```python
from build123d import *

# Parameters (mm, degrees)
IZIM1_W                     = 110
IZIM1_H                     = 70
Y_KSEKLIK_EKSTR_ZYON1_DEPTH = 2
IZIM2_W                     = 110
IZIM2_H                     = 70
Y_KSEKLIK_EKSTR_ZYON2_DEPTH = 50
IZIM3_R                     = 5.5
KES_EKSTR_ZYON1_DEPTH       = 13
IZIM4_R                     = 2.5
IZIM4_W                     = 15
IZIM4_H                     = 9
KES_EKSTR_ZYON2_DEPTH       = 13
IZIM5_R                     = 1.85
KES_EKSTR_ZYON3_DEPTH       = 67


with BuildPart() as part:
    # Çizim1 → Yükseklik-Ekstrüzyon1 (new body)
    with BuildSketch(Plane(origin=(0, 0, 0), x_dir=(1, 0, 0), z_dir=(0, 1, 0))):
        Rectangle(IZIM1_W, IZIM1_H)
    extrude(amount=Y_KSEKLIK_EKSTR_ZYON1_DEPTH)

    # Çizim2 → Yükseklik-Ekstrüzyon2 (add)
    with BuildSketch(Plane(origin=(0, 2, 0), x_dir=(1, 0, 0), z_dir=(0, 1, 0))):
        Rectangle(IZIM2_W, IZIM2_H)
        with BuildLine():
            Line((-48, -33.727272727), (48, -33.727272727))
            ThreePointArc((48, -33.727272727), (49.464466094, -30.191738821), (53, -28.727272727))
            Line((53, -28.727272727), (53, 28.727272727))
            ThreePointArc((53, 28.727272727), (49.464466094, 30.191738821), (48, 33.727272727))
            Line((48, 33.727272727), (-48, 33.727272727))
            ThreePointArc((-48, 33.727272727), (-49.464466094, 30.191738821), (-53, 28.727272727))
            Line((-53, 28.727272727), (-53, -28.727272727))
            ThreePointArc((-53, -28.727272727), (-49.464466094, -30.191738821), (-48, -33.727272727))
        make_face(mode=Mode.SUBTRACT)
    extrude(amount=Y_KSEKLIK_EKSTR_ZYON2_DEPTH)

    # Çizim3 → Kes-Ekstrüzyon1 (cut)
    with BuildSketch(Plane.ZY.offset(55)):
        with Locations((21.688585695, 26)):
            Circle(IZIM3_R)
    extrude(amount=-KES_EKSTR_ZYON1_DEPTH, mode=Mode.SUBTRACT)

    # Çizim4 → Kes-Ekstrüzyon2 (cut)
    with BuildSketch(Plane.ZY.offset(55)):
        with Locations((3.094292848, 26)):
            Circle(IZIM4_R)
        with Locations((-17.5, 30.5)):
            Rectangle(IZIM4_W, IZIM4_H)
    extrude(amount=-KES_EKSTR_ZYON2_DEPTH, mode=Mode.SUBTRACT)

    # Çizim5 → Kes-Ekstrüzyon3 (cut)
    with BuildSketch(Plane(origin=(0, 52, 0), x_dir=(1, 0, 0), z_dir=(0, 1, 0))):
        with Locations(Location((-52.232233047, 32.595869411, 0), (0, 0, 270))):
            Circle(IZIM5_R)
        with Locations(Location((52.232233047, 32.595869411, 0), (0, 0, 270))):
            Circle(IZIM5_R)
        with Locations(Location((52.232233047, -32.595869411, 0), (0, 0, 270))):
            Circle(IZIM5_R)
        with Locations(Location((-52.232233047, -32.595869411, 0), (0, 0, 270))):
            Circle(IZIM5_R)
    extrude(amount=-KES_EKSTR_ZYON3_DEPTH, mode=Mode.SUBTRACT)


solid = part.part
```
The model under review builds one solid part; all positions refer to its coordinate system, in mm. A direction names the side the tool comes from. Round coordinates to 2 decimals unless told otherwise and drop trailing zeros. Loops run counter-clockwise (first coordinate to the right, second up) from the corner with the lowest first, then second, coordinate; pieces in that order, holes last. Notation, with made-up numbers: (59, 32.5) - (116, 32.5) arc R32 ccw to (116, 63.5) - close; hole circle Ø1 at (-6.5, -34). An arc over 180 degrees is marked (long way). Use a Markdown table: item, result. Add a question column.
Q1. Add section B-B (x = -4.5). State the section outline as (y, z) points.
Q2. Add section C-C (y = 17). State the section outline as (x, z) points.
Q3. Add section A-A (z = 13). State the section outline as (x, y) points, plus the area to 3 significant figures.
Q4. For probe 1 along X at (y, z) = (32, 8.5); probe 2 along Z at (x, y) = (-15.5, 42); probe 3 along Y at (x, z) = (37, -18.5), list the stretches that pass through material, from the lowest coordinate up.
Q5. Machinability: for faces 4 (the face through (-54.014, 29.717, 17.635)), 5 (the face through (55, 26, 0)), 6 (the face through (-49.504, 26.65, 30.153)), which of the approach directions +Z, -Z, +X, -X, +Y, -Y give a long, thin tool a straight path to every point of the face, cutting with its end or side? Answer none if there is none.
Q6. The part is to be moulded in two halves that separate along Z. For faces 1 (the face through (-1, 0, 0)), 2 (the face through (-1, 26, -35)), 3 (the face through (53.48, 26.36, 31.23)), say which applies: pulls with the +Z half, pulls with the -Z half, needs draft (parallel to the pull), parting line crosses it, or undercut.
Q7. Insertion check: pin 1 Ø20 at (x, z) = (-2, 6.5) entering from +Y; pin 2 Ø3 at (x, z) = (-52.23, 32.6) entering from +Y; pin 3 Ø4.5 at (y, z) = (26, 3.09) entering from -X. Each pin has a flat end and moves straight along its axis. Give the tip position at first contact, or say it passes through.
Worked answers:
| question | item | result |
|---|---|---|
| 1 | outline | (0, -35) - (52, -35) - (52, -33.73) - (2, -33.73) - (2, 33.73) - (52, 33.73) - (52, 35) - (0, 35) - close |
| 2 | outline | (-55, -35) - (55, -35) - (55, 35) - (-55, 35) - close; hole circle Ø3.7 at (-52.23, -32.6); hole circle Ø3.7 at (-52.23, 32.6); hole (-53, -28.73) arc R5 cw to (-48, -33.73) - (48, -33.73) arc R5 cw to (53, -28.73) - (53, 28.73) arc R5 cw to (48, 33.73) - (-48, 33.73) arc R5 cw to (-53, 28.73) - close; hole circle Ø3.7 at (52.23, -32.6); hole circle Ø3.7 at (52.23, 32.6) |
| 3 | outline | (-55, 0) - (55, 0) - (55, 52) - (53, 52) - (53, 2) - (-53, 2) - (-53, 52) - (-55, 52) - close |
| 3 | area | 420 mm² |
| 4 | probe 1 | -55 to -53, 53 to 55 |
| 4 | probe 2 | -35 to -33.73, 33.73 to 35 |
| 4 | probe 3 | 0 to 2 |
| 5 | face 4 | -X |
| 5 | face 5 | +Z, -Z, +X, +Y, -Y |
| 5 | face 6 | +Y |
| 6 | face 1 | needs draft |
| 6 | face 2 | pulls with the -Z half |
| 6 | face 3 | undercut |
| 7 | pin 1 | y = 2 |
| 7 | pin 2 | through |
| 7 | pin 3 | x = 53 |
